```python
from build123d import *

# Parameters (mm, degrees)
F1_DEPTH    = 15.24
F2_T1_DEPTH = 217.8918149653
F2_T3_DEPTH = 128.5071697417
F2_T6_ANGLE = 90
F3_R        = 5.08
F4_R        = 6.3991299939
F5_DEPTH    = 43.18
F5_TAPER    = -4


# Not quite as in the source:
# - a fillet or chamfer that OpenCascade refuses, or shapes differently, is made with other operations: its cross-section is extruded or revolved along the edge and cut away or added


with BuildPart() as f1:
    # F0 (on Top) → F1 (new body)
    with BuildSketch(Plane.XY):
        with BuildLine():
            Line((120.7355335355, 76.0432109237), (-31.8355335355, 76.0432109237))
            ThreePointArc((-31.8355335355, 76.0432109237), (-94.697326383, 50.0050037712), (-120.7355335355, -12.8567890763))
            Line((-120.7355335355, -12.8567890763), (-120.7355335355, -76.0432109237))
            Line((-120.7355335355, -76.0432109237), (120.7355335355, -76.0432109237))
            Line((120.7355335355, -76.0432109237), (120.7355335355, 76.0432109237))
        make_face()
    extrude(amount=F1_DEPTH)

    # F2: chamfer of 25.4 on 1 edges, made by hand

    # F2_s2 → F2_t1 (cut)
    with BuildSketch(Plane.YZ.offset(-31.8355335355)):
        Polygon((76.0432109237, -10.16), (50.6432109237, 15.24), (76.0432109237, 15.24), align=None)
    extrude(amount=F2_T1_DEPTH, mode=Mode.SUBTRACT)

    # F2_s4 → F2_t3 (cut)
    with BuildSketch(Plane.XZ.offset(12.8567890763)):
        Polygon((-120.7355335355, -10.16), (-95.3355335355, 15.24), (-120.7355335355, 15.24), align=None)
    extrude(amount=F2_T3_DEPTH, mode=Mode.SUBTRACT)

    # F2_s5 → F2_t6 (revolve, cut)
    with BuildSketch(Plane.YZ.offset(-31.8355335355)):
        Polygon((76.0432109237, -10.16), (50.6432109237, 15.24), (76.0432109237, 15.24), align=None)
    revolve(axis=Axis((-31.8355335355, -12.8567890763, 15.24), (0, 0, 1)), revolution_arc=F2_T6_ANGLE, mode=Mode.SUBTRACT)

    # F3
    f3_edges = [f1.edges().sort_by_distance(p)[0] for p in [
        (12.7, -76.043211, 15.24),
    ]]
    fillet(f3_edges, radius=F3_R)

    # F4 (on face) → F5 (join)
    with BuildSketch(Plane.YZ.offset(120.7355335355)):
        with Locations((-12.1188843623, 7.419291418)):
            Circle(F4_R)
    extrude(amount=F5_DEPTH, taper=F5_TAPER)


solid = f1.part
```
The model under review builds one solid part; all positions refer to its coordinate system, in mm. Round coordinates to 2 decimals unless told otherwise and drop trailing zeros. Write each loop counter-clockwise with the first axis right and the second up, starting at its lowest first coordinate (ties: lowest second). Pieces come first, ordered by that corner, then holes. Notation, with made-up numbers: M 86.25,28 L 132.25,28 A20 ccw 132.25,62 Z; hole C -39.5,-36.75 d5. An arc over 180 degrees is marked long. Use CSV: the item, a comma, the result in double quotes. Start each with the question number.
(1) The part is to be moulded in two halves that separate along X. For faces 1 (the face through (3, -76.043, 5)), 2 (the face through (142.63, -7.86, 14.11)), 3 (the face through (-103.062, -44.008, 7.513)), say which applies: +X half, -X half, draft (parallel to the pull), parting line (faces both ways), or undercut.
(2) Clearance check with flat-ended pins moving along their axes: P1, Ø2, axis at y = -57, z = 4, coming from the -X side; P2, Ø6, axis at x = 135, z = 13, coming from the +Y side; P3, Ø10, axis at y = 50, z = 14, coming from the +X side. State where each tip first meets the part, or that it passes through.
(3) We need section A-A, the plane y = -25.5. State the section outline as (x, z) points, then the cut area to 3 significant figures.
(4) For line 1 along Z through (x, y) = (105, -58.5); line 2 along X through (y, z) = (-17.5, 8); line 3 along X through (y, z) = (-23, 2.75), list the stretches that pass through material, from the lowest coordinate up.
(5) We need section B-B, the plane x = 25. State the section outline as (y, z) points.
Findings:
1,face 1,"draft"
1,face 2,"undercut"
1,face 3,"-X half"
2,P1,"x = -107.58"
2,P2,"y = -5.17"
2,P3,"x = 120.74"
3,outline,"M -110.58,0 L 120.74,0 L 120.74,15.24 L -95.34,15.24 Z"
3,area,"3,410 mm^2"
4,line 1,"0 to 15.24"
4,line 2,"-102.58 to 163.92"
4,line 3,"-107.83 to 120.74"
5,outline,"M -76.04,0 L 65.88,0 L 50.64,15.24 L -70.96,15.24 A5.08 ccw -76.04,10.16 Z"
